For this review, take the finished solid that the model builds, in its own axes (mm). A direction names the side the tool comes from. Round coordinates to 2 decimals unless told otherwise and drop trailing zeros. Loops run counter-clockwise (first coordinate to the right, second up) from the corner with the lowest first, then second, coordinate; pieces in that order, holes last.
1. Clearance check with flat-ended pins moving along their axes: pin 1 Ø2 at (y, z) = (-4, 87) entering from +X; pin 2 Ø1.5 at (x, y) = (-5, 1) entering from -Z; pin 3 Ø12 at (y, z) = (-7, 149) entering from -X. State where each tip first meets the part, or that it passes through.
2. Draft analysis for pull direction X (two halves, no side actions). For faces 1 (the flat face through (0, 0, 8)), 2 (the cylindrical face through (-2.17, -9.76, 86.78)), 3 (the flat face through (0, 0, -10)), state which applies: released by +X, released by -X, zero draft, split by the parting line, or undercut.
3. To check wall thickness, follow line 1 along Y through (x, z) = (0, 70); line 2 along X through (y, z) = (0.5, 142.5); line 3 along Y through (x, z) = (0, 174.3). State the ranges of each line that lie inside material, in increasing order.
4. Consider section C-C on z = 129. State the section outline as (x, y) points, then the cut area to 3 significant figures.
5. Consider section A-A on y = 0. State the section outline as (x, z) points, then the cut area to 3 significant figures.
6. Tool access review of faces 4 (the cylindrical face through (6.466, -2.681, 91.148)), 5 (the cylindrical face through (-6, 0, 174)), 6 (the cylindrical face through (0.867, -3.905, -4.93)): name each direction out of +Z, -Z, +X, -X, +Y, -Y from which nothing blocks a thin tool from reaching the whole face with its end or side.
from build123d import *

# Parameters (mm, degrees)
SKETCH_1_R          = 10
EXTRUDE_1_DEPTH     = 175
SKETCH_2_R          = 7
CUT_EXTRUDE_1_DEPTH = 167
SKETCH_3_R          = 4
EXTRUDE_2_DEPTH     = 10
CHAMFER_1_SIZE      = 1
SKETCH_4_R          = 7
SKETCH_4_R_2        = 6
EXTRUDE_3_DEPTH     = 3


with BuildPart() as part:
    # 草图1 → 凸台-拉伸1 (new body)
    with BuildSketch(Plane.XY):
        Circle(SKETCH_1_R)
    extrude(amount=EXTRUDE_1_DEPTH)

    # 草图2 → 切除-拉伸1 (cut)
    with BuildSketch(Plane.XY.offset(175)):
        Circle(SKETCH_2_R)
    extrude(amount=-CUT_EXTRUDE_1_DEPTH, mode=Mode.SUBTRACT)

    # 草图3 → 凸台-拉伸2 (add)
    with BuildSketch(Plane(origin=(0, 0, 0), x_dir=(-1, 0, 0), z_dir=(0, 0, -1))):
        Circle(SKETCH_3_R)
    extrude(amount=EXTRUDE_2_DEPTH)

    # 倒角1
    chamfer_1_edges = [part.edges().sort_by_distance(p)[0] for p in [
        (-10, 0, 0),
    ]]
    chamfer(chamfer_1_edges, length=CHAMFER_1_SIZE)

    # 草图4 → 凸台-拉伸3 (add)
    with BuildSketch(Plane.XY.offset(175)):
        Circle(SKETCH_4_R)
        Circle(SKETCH_4_R_2, mode=Mode.SUBTRACT)
    extrude(amount=-EXTRUDE_3_DEPTH)


solid = part.part
Resolved:
1. pin 1: stops at x = 9.54
1. pin 2: stops at z = 0
1. pin 3: stops at x = -9.95
2. face 1: undercut
2. face 2: split by the parting line
2. face 3: zero draft
3. line 1: y = -10 to -7, 7 to 10
3. line 2: x = -9.99 to -6.98, 6.98 to 9.99
3. line 3: y = -10 to -6, 6 to 10
4. outline: circle Ø20 at (0, 0); hole circle Ø14 at (0, 0)
4. area: 160 mm2
5. outline: (-10, 1) - (-9, 0) - (-4, 0) - (-4, -10) - (4, -10) - (4, 0) - (9, 0) - (10, 1) - (10, 175) - (6, 175) - (6, 172) - (7, 172) - (7, 8) - (-7, 8) - (-7, 172) - (-6, 172) - (-6, 175) - (-10, 175) - close
5. area: 1,250 mm2
6. face 4: none
6. face 5: +Z
6. face 6: -Z
